from build123d import *

# Parameters (mm, degrees)
SKETCH1_R           = 5
BOSS_EXTRUDE1_DEPTH = 5
FILLET1_R           = 15
SKETCH2_R           = 1.25
CUT_EXTRUDE1_DEPTH  = 42.003048667


with BuildPart() as part:
    # Sketch1 → Boss-Extrude1 (new body)
    with BuildSketch(Plane(origin=(0, 0, 0), x_dir=(1, 0, 0), z_dir=(0, 1, 0))):
        with BuildLine():
            ThreePointArc((5, 0), (-0.30604892, -4.990624616), (-4.962533624, 0.610950109))
            Line((-4.962533624, 0.610950109), (-7.5, -20))
            Line((-7.5, -20), (-7.5, -40))
            Line((-7.5, -40), (7.5, -40))
            Line((7.5, -40), (7.5, -20))
            Line((7.5, -20), (4.962533624, 0.610950109))
            ThreePointArc((4.962533624, 0.610950109), (4.990624616, 0.30604892), (5, 0))
        make_face()
        Circle(SKETCH1_R)
    extrude(amount=BOSS_EXTRUDE1_DEPTH)

    # Fillet1
    fillet1_edges = [part.edges().sort_by_distance(p)[0] for p in [
        (7.5, 2.5, 20),
        (-7.5, 2.5, 20),
    ]]
    fillet(fillet1_edges, radius=FILLET1_R)

    # Sketch2 → Cut-Extrude1 (cut, through all)
    with BuildSketch(Plane(origin=(0, 5, 0), x_dir=(1, 0, 0), z_dir=(0, 1, 0))):
        with Locations(Location((0, 0, 0), (0, 0, 270))):
            Circle(SKETCH2_R)
        with Locations(Location((0, -20, 0), (0, 0, 270))):
            Circle(SKETCH2_R)
    extrude(amount=-CUT_EXTRUDE1_DEPTH, mode=Mode.SUBTRACT)


solid = part.part
Verification items for the finished model (mm, model axes). Round coordinates to 2 decimals unless told otherwise and drop trailing zeros. Order: outer loops, then holes, each group sorted by start corner. A loop starts at its lowest first (then second) coordinate and runs counter-clockwise, first axis right, second up. Notation, with made-up numbers: (43.25, 54) -> (61.25, 54) arc R20 cw to (61.25, 88) -> close; hole circle Ø7 at (-1, -25). An arc over 180 degrees is marked (long way). Put each result on its own line as item: value.
1) Section check C-C (z = 0). Record the cut outline in (x, y), then the cut area to 3 significant figures.
Final values:
outline: (-5.04, 0) -> (-1.25, 0) -> (-1.25, 5) -> (-5.04, 5) -> close; (1.25, 0) -> (5.04, 0) -> (5.04, 5) -> (1.25, 5) -> close
area: 37.9 mm^2
2) Section check B-B (y = 4.25). Record the cut outline in (x, z).
Final values:
outline: (-7.5, 20.92) arc R15 ccw to (-7.39, 19.09) -> (-4.96, -0.61) arc R5 ccw to (4.96, -0.61) -> (7.39, 19.09) arc R15 ccw to (7.5, 20.92) -> (7.5, 40) -> (-7.5, 40) -> close; hole circle Ø2.5 at (0, 0); hole circle Ø2.5 at (0, 20)
3) Mould release check, pull along X, two halves, no side actions. Record for faces 1 (the cylindrical face through (7.473, 2.535, 20.015)), 2 (the flat face through (0, 2, 40)), 3 (the cylindrical face through (-1.22, 2.54, -0.27)), 4 (the flat face through (-6.16, 2.46, 9.1)): +X half, -X half, draft (parallel to the pull), parting line (faces both ways), or undercut.
Final values:
face 1: +X half
face 2: draft
face 3: undercut
face 4: -X half
4) Material ranges on line 1 (Z direction, x = -0.5, y = 1.4); line 2 (Z direction, x = 1, y = 2); line 3 (X direction, y = 1.5, z = 20), recorded low to high.
Final values:
line 1: z = -4.97 to -1.15, 1.15 to 18.85, 21.15 to 40
line 2: z = -4.9 to -0.75, 0.75 to 19.25, 20.75 to 40
line 3: x = -7.47 to -1.25, 1.25 to 7.47
5) Depth check by flat-ended pin: pin 1 (1 mm diameter, centred on y = 1, z = 2, fed in from -X). Enter the tip coordinate at first touch or a pass-through.
Final values:
pin 1: stops at x = -5.35
6) Section check A-A (x = 0). Record the cut outline in (y, z).
Final values:
outline: (0, -5) -> (5, -5) -> (5, -1.25) -> (0, -1.25) -> close; (0, 1.25) -> (5, 1.25) -> (5, 18.75) -> (0, 18.75) -> close; (0, 21.25) -> (5, 21.25) -> (5, 40) -> (0, 40) -> close
7) Section check D-D (z = 20). Record the cut outline in (x, y), then the cut area to 3 significant figures.
Final values:
outline: (-7.47, 0) -> (-1.25, 0) -> (-1.25, 5) -> (-7.47, 5) -> close; (1.25, 0) -> (7.47, 0) -> (7.47, 5) -> (1.25, 5) -> close
area: 62.2 mm^2
